Here's how the part is built. I have some questions about the finished solid (model axes, mm). A direction names the side the tool comes from. Round coordinates to 2 decimals unless told otherwise and drop trailing zeros. Order: outer loops, then holes, each group sorted by start corner. A loop starts at its lowest first (then second) coordinate and runs counter-clockwise, first axis right, second up. Notation, with made-up numbers: (-23, 22) -> (35, 22) arc R37 cw to (35, 58) -> close; hole circle Ø3 at (-30, 48.5). An arc over 180 degrees is marked (long way). One line per item, written item: value.
```python
from build123d import *

# Parameters (mm, degrees)
EXTRUDE_1_DEPTH       = 800
EXTRUDE_2_DEPTH       = 300
MIRROR_3_COPY_1_DEPTH = 300
MIRROR_3_COPY_2_DEPTH = 300


with BuildPart() as part:
    # 草图1 → 凸台-拉伸1 (new body)
    with BuildSketch(Plane(origin=(0, 0, 0), x_dir=(1, 0, 0), z_dir=(0, 1, 0))):
        with BuildLine():
            Line((0, 705), (0, 680))
            ThreePointArc((0, 680), (446.120139714, 513.202514551), (673.382286744, 94.637708653))
            Line((673.382286744, 94.637708653), (698.138988463, 98.117036177))
            ThreePointArc((698.138988463, 98.117036177), (462.521615438, 532.070254057), (0, 705))
        make_face()
    extrude(amount=EXTRUDE_1_DEPTH)

    # 草图2 → 凸台-拉伸2 (add)
    with BuildSketch(Plane(origin=(0, 400, 0), x_dir=(1, 0, 0), z_dir=(0, 1, 0))):
        Polygon((698.138988463, 98.117036177), (673.382286744, 94.637708653), (676.691143372, 47.318854326), (700.56509889, 63.422040654), align=None)
    extrude_2 = extrude(amount=-EXTRUDE_2_DEPTH)

    # 镜向1: 凸台-拉伸2 across plane
    add(extrude_2.mirror(Plane(origin=(446.120139714, 800, -513.202514551), x_dir=(-0.6560590289905062, 0, 0.754709580222773), z_dir=(-0.7547095802227732, 0, -0.656059028990506))))

    # 镜向2: 凸台-拉伸2 across plane
    add(extrude_2.mirror(Plane.ZX.offset(400)))

    # 镜向3 copy 1 sketch → 镜向3 copy 1 (add)
    with BuildSketch(Plane(origin=(0, 400, 0), x_dir=(-0.13917310096006918, 0, -0.99026806874157), z_dir=(0, -1, 0))):
        Polygon((698.138988463, 98.117036177), (673.382286744, 94.637708653), (676.691143372, 47.318854326), (700.56509889, 63.422040654), align=None)
    extrude(amount=-MIRROR_3_COPY_1_DEPTH)

    # 镜向3 copy 2 sketch → 镜向3 copy 2 (add)
    with BuildSketch(Plane(origin=(0, 400, 0), x_dir=(-0.13917310096006918, 0, -0.99026806874157), z_dir=(0, 1, 0))):
        Polygon((698.138988463, -98.117036177), (673.382286744, -94.637708653), (676.691143372, -47.318854326), (700.56509889, -63.422040654), align=None)
    extrude(amount=-MIRROR_3_COPY_2_DEPTH)


solid = part.part
```
Q1. If we mould it in two halves opening along X, with no side actions, what happens to faces 1 (the face through (-18, 700, -691)), 2 (the face through (699.37, 395.8, -80.53)), 3 (the face through (-23.33, 395.8, -678.37)), 4 (the face through (-41.095, 395.8, -689.451))? For each: pulls with the +X half, pulls with the -X half, needs draft (parallel to the pull), parting line crosses it, or undercut.
Answers:
face 1: needs draft
face 2: pulls with the +X half
face 3: undercut
face 4: pulls with the -X half
Q2. I want a section at C-C on z = -261. Write out the boundary of the cut face in (x, y), then the cut area to 3 significant figures.
Answers:
outline: (627.92, 0) -> (654.91, 0) -> (654.91, 800) -> (627.92, 800) -> close
area: 21,600 mm2
Q3. Which directions (+Z, -Z, +X, -X, +Y, -Y) give clear straight access to the entire face, cutting with the end or side of a thin tool? Please do faces 5 (the face through (0, 49, -693)), 6 (the face through (685.587, 49.3, -96.353)), 7 (the face through (685.587, 749.3, -96.353)).
Answers:
face 5: +Z, -Z, -X, -Y
face 6: +Z, +X, -Y
face 7: +Z, +X, +Y
Q4. I want a section at A-A on y = 435. Write out the boundary of the cut face in (x, z) (3 decimals).
Answers:
outline: (-47.319, -676.691) -> (-34.695, -702.574) -> (0, -705) arc R705 ccw to (698.139, -98.117) -> (700.565, -63.422) -> (676.691, -47.319) -> (673.382, -94.638) arc R680 cw to (0, -680) -> close
Q5. I want a section at B-B on x = 626. Write out the boundary of the cut face in (y, z).
Answers:
outline: (0, -324.27) -> (800, -324.27) -> (800, -265.56) -> (0, -265.56) -> close
Q6. I need wall thicknesses on line 1 along Z through (x, y) = (8.5, 588); line 2 along Z through (x, y) = (1.5, 404.5); line 3 along X through (y, z) = (523, -521.5). Which ranges of each line are inside material? Lowest first, please.
Answers:
line 1: -704.95 to -679.95
line 2: -705 to -680
line 3: 436.39 to 474.41
Q7. For P1, Ø2, axis at y = 665.5, z = -581, coming from the -X side; P2, Ø21.5, axis at x = 681.5, z = -64, coming from the -Y side; P3, Ø3, axis at x = 226.5, y = 518, coming from the -Z side, each with a flat end and sliding along its axis, tell me the tip position at first contact or that it passes through.
Answers:
P1: x = 351.68
P2: y = 100
P3: z = -668.13
